Verification items for the finished model (mm, model axes). Coordinates: 2 decimals unless noted, no trailing zeros. Write each loop counter-clockwise with the first axis right and the second up, starting at its lowest first coordinate (ties: lowest second). Pieces come first, ordered by that corner, then holes.
```python
from build123d import *

# Parameters (mm, degrees)
ESQUISSE1_W        = 230
ESQUISSE1_H        = 170
BOSS_EXTRU_1_DEPTH = 3
ESQUISSE2_W        = 30
ESQUISSE2_H        = 3
BOSS_EXTRU_6_DEPTH = 3
ESQUISSE4_W        = 3
ESQUISSE4_H        = 30
BOSS_EXTRU_7_DEPTH = 3


with BuildPart() as part:
    # Esquisse1 → Boss.-Extru.1 (new body)
    with BuildSketch(Plane.XY):
        with Locations((29.537157757, -23.076923077)):
            Rectangle(ESQUISSE1_W, ESQUISSE1_H)
    extrude(amount=BOSS_EXTRU_1_DEPTH)

    # Esquisse2 → Boss.-Extru.6 (add)
    with BuildSketch(Plane(origin=(0, 0, 0), x_dir=(-1, 0, 0), z_dir=(0, 0, -1))):
        with Locations((-129.537157757, 63.423076923)):
            Rectangle(ESQUISSE2_W, ESQUISSE2_H)
        with Locations((-69.537157757, 63.423076923)):
            Rectangle(ESQUISSE2_W, ESQUISSE2_H)
        with Locations((-9.537157757, 63.423076923)):
            Rectangle(ESQUISSE2_W, ESQUISSE2_H)
        with Locations((50.462842243, 63.423076923)):
            Rectangle(ESQUISSE2_W, ESQUISSE2_H)
        with Locations((50.462842243, -109.576923077)):
            Rectangle(ESQUISSE2_W, ESQUISSE2_H)
        with Locations((-129.537157757, -109.576923077)):
            Rectangle(ESQUISSE2_W, ESQUISSE2_H)
        with Locations((-69.537157757, -109.576923077)):
            Rectangle(ESQUISSE2_W, ESQUISSE2_H)
        with Locations((-9.537157757, -109.576923077)):
            Rectangle(ESQUISSE2_W, ESQUISSE2_H)
    extrude(amount=-BOSS_EXTRU_6_DEPTH)

    # Esquisse4 → Boss.-Extru.7 (add)
    with BuildSketch(Plane(origin=(0, 0, 0), x_dir=(-1, 0, 0), z_dir=(0, 0, -1))):
        with Locations((86.962842243, 46.923076923)):
            Rectangle(ESQUISSE4_W, ESQUISSE4_H)
        with Locations((86.962842243, -13.076923077)):
            Rectangle(ESQUISSE4_W, ESQUISSE4_H)
        with Locations((86.962842243, -73.076923077)):
            Rectangle(ESQUISSE4_W, ESQUISSE4_H)
        with Locations((-146.037157757, 46.923076923)):
            Rectangle(ESQUISSE4_W, ESQUISSE4_H)
        with Locations((-146.037157757, -13.076923077)):
            Rectangle(ESQUISSE4_W, ESQUISSE4_H)
        with Locations((-146.037157757, -73.076923077)):
            Rectangle(ESQUISSE4_W, ESQUISSE4_H)
    extrude(amount=-BOSS_EXTRU_7_DEPTH)


solid = part.part
```
1. Sectioned sample at B-B, the plane x = 45.5. Record the boundary of the cut face in (y, z), and give its area (3 significant figures).
2. Sectioned sample at A-A, the plane y = -37. Record the boundary of the cut face in (x, z).
3. Gauge pin test, flat ends, axial feed: P1, Ø0.9, axis at y = -109, z = 1, coming from the +X side; P2, Ø0.9, axis at x = 147, z = 1, coming from the +Y side; P3, Ø1.5, axis at y = -110, z = 2, coming from the -X side. Record the tip position at first contact, or that the pin passes through.
4. Material ranges on L1, parallel to Y at x = -69.5, z = 2.7; L2, parallel to X at y = -44, z = 2, recorded low to high.
Outcome:
1. outline: (-108.08, 0) - (61.92, 0) - (61.92, 3) - (-108.08, 3) - close
1. area: 510 mm2
2. outline: (-85.46, 0) - (144.54, 0) - (144.54, 3) - (-85.46, 3) - close
3. P1: stops at x = 144.54
3. P2: stops at y = 61.92
3. P3: stops at x = -65.46
4. L1: y = -108.08 to 61.92
4. L2: x = -85.46 to 144.54
